Here's how the part is built. I have some questions about the finished solid (model axes, mm). A direction names the side the tool comes from. Round coordinates to 2 decimals unless told otherwise and drop trailing zeros. Order: outer loops, then holes, each group sorted by start corner. A loop starts at its lowest first (then second) coordinate and runs counter-clockwise, first axis right, second up. Notation, with made-up numbers: (24.25, 34) - (39.25, 34) arc R19 ccw to (39.25, 50) - close; hole circle Ø9 at (63.5, -16). An arc over 180 degrees is marked (long way). Answer as a JSON object with one key per item and string values.
Solid Edge part; units mm, degrees
sketch "Sketch1" plane through (0, 0, 0) normal (0, 0, 1) x (1, 0, 0)
  circle A0 centre (0, 0) radius 70
  circle A1 centre (0, 0) radius 35
extrude "Protrusion1" add sketch "Sketch1" along normal blind 20
sketch "Sketch2" plane through (0, 0, 0) normal (0, 0, 1) x (1, 0, 0)
  circle A0 centre (0, 0) radius 35
  circle A1 centre (0, 0) radius 25
extrude "ExtrudedProtrusion_12" add sketch "Sketch2" along normal blind 90
sketch "Sketch3" plane through (0, 0, 20) normal (0, 0, 1) x (1, 0, 0)
  circle A0 centre (-50, 0) radius 5
  circle A1 centre (0, 50) radius 5
  circle A2 centre (50, 0) radius 5
  circle A3 centre (0, -50) radius 5
extrude "Cutout1" cut sketch "Sketch3" against normal up to vertex (20 mm away)
1. Thinking about a two-plate mould opening in Y: for faces 3 (the face through (45, 0, 10)), 4 (the face through (-55.55, 42.594, 9.86)), 5 (the face through (-0.651, 54.957, 10.14)), 6 (the face through (-32, -15, 20)), which applies, pulls with the +Y half, pulls with the -Y half, needs draft (parallel to the pull), parting line crosses it, or undercut?
Responses:
{"face 3": "undercut", "face 4": "parting line crosses it", "face 5": "undercut", "face 6": "needs draft"}
2. Imagine slicing it at D-D (z = 15). List the corners of the cut face in (x, y) for me.
Responses:
{"outline": "circle Ø140 at (0, 0); hole circle Ø10 at (-50, 0); hole circle Ø50 at (0, 0); hole circle Ø10 at (0, -50); hole circle Ø10 at (0, 50); hole circle Ø10 at (50, 0)"}
3. Imagine slicing it at B-B (y = -19). List the corners of the cut face in (x, z) for me, plus the area to 3 significant figures.
Responses:
{"outline": "(-67.37, 0) - (-16.25, 0) - (-16.25, 90) - (-29.39, 90) - (-29.39, 20) - (-67.37, 20) - close; (16.25, 0) - (67.37, 0) - (67.37, 20) - (29.39, 20) - (29.39, 90) - (16.25, 90) - close", "area": "3,890 mm2"}
4. If I drill on L1, parallel to Y at x = 0, z = 38; L2, parallel to Z at x = -27, y = 55.5; L3, parallel to Y at x = 50, z = 14.5, over which ranges is the centre line in solid material (lowest first)? Write a range as [from, to].
Responses:
{"L1": "[-35, -25], [25, 35]", "L2": "[0, 20]", "L3": "[-48.99, -5], [5, 48.99]"}
5. For P1, Ø16, axis at x = -50, y = 0, coming from the +Z side; P2, Ø8, axis at x = 4.5, z = 79.5, coming from the +Y side; P3, Ø5, axis at x = -5.5, z = 17, coming from the +Y side; P4, Ø9, axis at x = 0, y = 50, coming from the -Z side, each with a flat end and sliding along its axis, tell me the tip position at first contact or that it passes through.
Responses:
{"P1": "z = 20", "P2": "y = 35", "P3": "y = 69.94", "P4": "through"}
6. Imagine slicing it at C-C (x = -22.5). List the corners of the cut face in (y, z) for me, plus the area to 3 significant figures.
Responses:
{"outline": "(-66.29, 0) - (-10.9, 0) - (-10.9, 90) - (-26.81, 90) - (-26.81, 20) - (-66.29, 20) - close; (10.9, 0) - (66.29, 0) - (66.29, 20) - (26.81, 20) - (26.81, 90) - (10.9, 90) - close", "area": "4,440 mm2"}
7. Imagine slicing it at A-A (x = 0). List the corners of the cut face in (y, z) for me, plus the area to 3 significant figures.
Responses:
{"outline": "(-70, 0) - (-55, 0) - (-55, 20) - (-70, 20) - close; (-45, 0) - (-25, 0) - (-25, 90) - (-35, 90) - (-35, 20) - (-45, 20) - close; (25, 0) - (45, 0) - (45, 20) - (35, 20) - (35, 90) - (25, 90) - close; (55, 0) - (70, 0) - (70, 20) - (55, 20) - close", "area": "2,800 mm2"}
8. For faces 1 (the face through (-28, 21, 55)), 2 (the face through (-24, 8, 90)), which set-ups out of +Z, -Z, +X, -X, +Y, -Y let a thin tool reach every point of the face, with its end or its side?
Responses:
{"face 1": "+Z", "face 2": "+Z, +X, -X, +Y, -Y"}
